Read the model definition and answer for the solid it produces. Units are mm, in the model's axes. Face numbers are marked on the shaded views. A direction names the side the tool comes from. Round coordinates to 2 decimals unless told otherwise and drop trailing zeros. Write each loop counter-clockwise with the first axis right and the second up, starting at its lowest first coordinate (ties: lowest second). Pieces come first, ordered by that corner, then holes. Notation, with made-up numbers: (21.25, -40) - (77.25, -40) arc R7 cw to (77.25, -28) - close; hole circle Ø2 at (-14.5, 76). An arc over 180 degrees is marked (long way). Use one line per item in the form item = value. Start each with the question number.
1) The part is cut by section D-D, the plane x = -5.5. Give the vertices of the cut face in (y, z) (3 decimals).
2) Each of these flat-tipped pins is pushed along its axis until it touches: pin 1 (1 mm diameter, centred on x = 6.5, y = -3.5, fed in from +Z); pin 2 (2 mm diameter, centred on x = -6.5, y = -1, fed in from +Z). Where does it stop, or does it pass through?
3) The part is cut by section B-B, the plane x = -0.75. Give the vertices of the cut face in (y, z), plus the area to 3 significant figures.
4) For the marked faces 1 and 2, determine the directions among +Z, -Z, +X, -X, +Y, -Y from which every point of the face is accessible in a straight line to the end or side of a thin tool.
5) Consider line 1 along Y through (x, z) = (-5.5, 0.5); line 2 along Y through (x, z) = (0.75, 3); line 3 along X through (y, z) = (-3, 0). Determine where each line is inside the solid, lowest interval first. Write a range as from..to.
6) The part is cut by section A-A, the plane z = 5. Give the vertices of the cut face in (x, y), plus the area to 3 significant figures.
7) The part is cut by section C-C, the plane y = -2. Give the vertices of the cut face in (x, z), plus the area to 3 significant figures.
8) For a pull along Y with two mould halves and no side action, classify the marked faces 3, 4 and 5 as released by +Y, released by -Y, zero draft, split by the parting line, or undercut.
Autodesk Inventor part; units mm, degrees
ref_plane "YZ Plane" through (0, 0, 0) normal (1, 0, 0) x (0, 1, 0)
ref_plane "XZ Plane" through (0, 0, 0) normal (0, 1, 0) x (-1, 0, 0)
ref_plane "XY Plane" through (0, 0, 0) normal (0, 0, 1) x (1, 0, 0)
sketch "Sketch1" plane through (0, 0, 0) normal (0, 0, 1) x (1, 0, 0)
  line L0 (-8.4582, 8.1026) -> (8.4582, 8.1026)
  line L1 (8.4582, 8.1026) -> (8.4582, -8.1026)
  line L2 (8.4582, -8.1026) -> (-8.4582, -8.1026)
  line L3 (-8.4582, -8.1026) -> (-8.4582, 8.1026)
  line L4 (0, 0) -> (0, 8.1026) construction
  line L5 (0, 0) -> (0, -8.1026) construction
  line L6 (0, 0) -> (-8.4582, 0) construction
  line L7 (0, 0) -> (8.4582, 0) construction
  dimension "d0" = 16.9164
  dimension "d1" = 16.2052
extrude "Extrusion1" add sketch "Sketch1" along normal mid plane 16.8656
sketch "Sketch2" plane through (0, 0, 8.4328) normal (0, 0, 1) x (1, 0, 0)
  line L0 (8.4582, 8.1026) -> (8.4582, -8.1026)
  line L1 (-8.4582, 8.1026) -> (8.4582, 8.1026)
  line L2 (-8.4582, -8.1026) -> (-8.4582, 8.1026)
  line L3 (8.4582, -8.1026) -> (-8.4582, -8.1026)
  line L4 (-8.2042, -2.54) -> (-8.2042, 2.54)
  line L5 (-8.2042, 2.54) -> (-4.3942, 2.54)
  line L6 (-4.3942, 2.54) -> (-4.3942, 6.731)
  line L7 (-4.3942, 6.731) -> (2.8702, 6.731)
  line L8 (2.8702, 6.731) -> (2.8702, -6.731)
  line L9 (2.8702, -6.731) -> (-4.3942, -6.731)
  line L10 (-4.3942, -6.731) -> (-4.3942, -2.54)
  line L11 (-4.3942, -2.54) -> (-8.2042, -2.54)
  line L12 (0, 8.1026) -> (0, -8.1026) construction
  line L13 (-8.4582, 0) -> (8.4582, 0) construction
  dimension "d4" = 13.462
  dimension "d5" = 0.254
  dimension "d6" = 3.81
  dimension "d7" = 5.08
  dimension "d8" = 5.588
extrude "Extrusion2" cut sketch "Sketch2" against normal blind 10.16 contours L4 L5 L6 L7 L8 L9 L10 L11
sketch "Sketch3" plane through (0, 0, 8.4328) normal (0, 0, 1) x (1, 0, 0)
  line L0 (-8.2042, 2.54) -> (-4.3942, 2.54)
  line L1 (-4.3942, 2.54) -> (-4.3942, 6.731)
  line L2 (-4.3942, 6.731) -> (2.8702, 6.731)
  line L3 (-7.0612, 6.731) -> (-5.0292, 6.731)
  line L4 (-5.0292, 6.731) -> (-5.0292, 3.175)
  line L5 (-5.0292, 3.175) -> (-7.0612, 3.175)
  line L6 (-7.0612, 3.175) -> (-7.0612, 6.731)
  dimension "d11" = 0.635
  dimension "d12" = 0.635
  dimension "d13" = 2.032
extrude "Extrusion3" add sketch "Sketch3" along normal blind 0.0254
mirror "Mirror1" about plane through (0, 0, 0) normal (0, 1, 0) of "Extrusion3"
properties part number "cRIO-FRC CAT5" material "ABS Plastic"
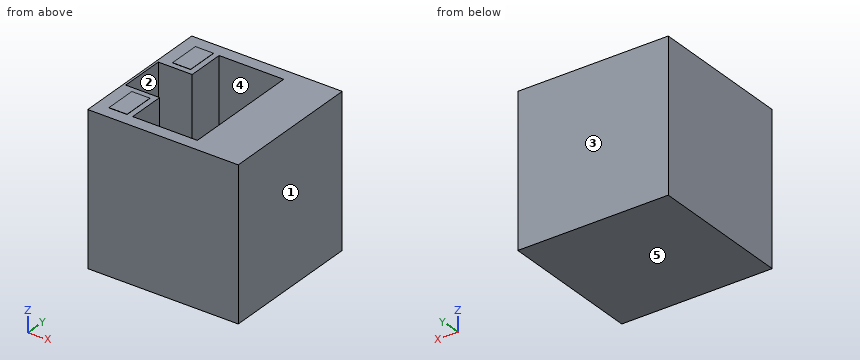
Geometry results:
q1.outline = (-8.103, -8.433) - (8.103, -8.433) - (8.103, 8.433) - (6.731, 8.433) - (6.731, 8.458) - (3.175, 8.458) - (3.175, 8.433) - (2.54, 8.433) - (2.54, -1.727) - (-2.54, -1.727) - (-2.54, 8.433) - (-3.175, 8.433) - (-3.175, 8.458) - (-6.731, 8.458) - (-6.731, 8.433) - (-8.103, 8.433) - close
q2.pin_1 = 8.43
q2.pin_2 = -1.73
q3.outline = (-8.1, -8.43) - (8.1, -8.43) - (8.1, 8.43) - (6.73, 8.43) - (6.73, -1.73) - (-6.73, -1.73) - (-6.73, 8.43) - (-8.1, 8.43) - close
q3.area = 137 mm2
q4.face_1 = +Z, -Z, +X, +Y, -Y
q4.face_2 = +Z
q5.line_1 = -8.1..-2.54, 2.54..8.1
q5.line_2 = -8.1..-6.73, 6.73..8.1
q5.line_3 = -8.46..-4.39, 2.87..8.46
q6.outline = (-8.46, -8.1) - (8.46, -8.1) - (8.46, 8.1) - (-8.46, 8.1) - close; hole (-8.2, -2.54) - (-4.39, -2.54) - (-4.39, -6.73) - (2.87, -6.73) - (2.87, 6.73) - (-4.39, 6.73) - (-4.39, 2.54) - (-8.2, 2.54) - close
q6.area = 157 mm2
q7.outline = (-8.46, -8.43) - (8.46, -8.43) - (8.46, 8.43) - (2.87, 8.43) - (2.87, -1.73) - (-8.2, -1.73) - (-8.2, 8.43) - (-8.46, 8.43) - close
q7.area = 173 mm2
q8.face_3 = released by +Y
q8.face_4 = undercut
q8.face_5 = zero draft
